from build123d import *

# Parameters (mm, degrees)
SKETCH2_W   = 60
SKETCH2_H   = 60
SKETCH2_W_2 = 50
SKETCH2_H_2 = 50


with BuildPart() as part:
    # Sweep1: sweep along a path in Sketch1
    with BuildLine(Plane.XY) as sweep1_path:
        Line((330, 0), (330, 1500))
        Line((330, 1500), (185.671137026, 1698.283381924))
        Line((185.671137026, 1698.283381924), (0, 1698.283381924))
    # Sketch2 → Sweep1 (sweep)
    with BuildSketch(Plane(origin=(0, 0, 0), x_dir=(1, 0, 0), z_dir=(0, 1, 0))):
        with Locations((330, 0)):
            Rectangle(SKETCH2_W, SKETCH2_H)
        with Locations((330, 0)):
            Rectangle(SKETCH2_W_2, SKETCH2_H_2, mode=Mode.SUBTRACT)
    sweep1 = sweep(path=sweep1_path.line, transition=Transition.RIGHT)

    # Mirror1: Sweep1 across plane
    add(sweep1.mirror(Plane(origin=(0, 0, 0), x_dir=(0, 0, 1), z_dir=(1, 0, 0))))


solid = part.part
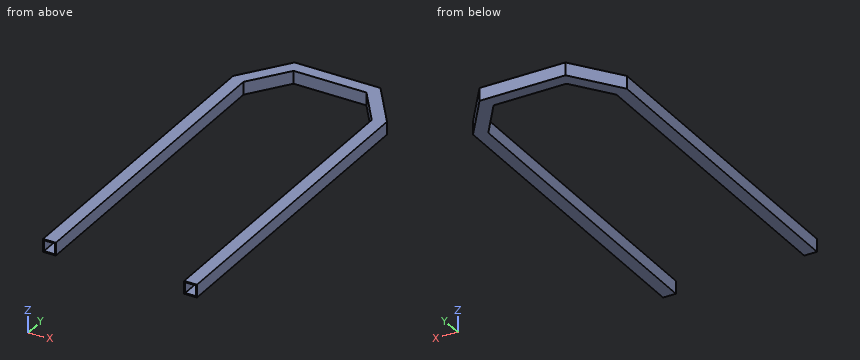
Here's how the part is built. I have some questions about the finished solid (model axes, mm). Round coordinates to 2 decimals unless told otherwise and drop trailing zeros. Write each loop counter-clockwise with the first axis right and the second up, starting at its lowest first coordinate (ties: lowest second). Pieces come first, ordered by that corner, then holes.
1. Suppose I cut it at D-D (x = 256.5). List the corners of the cut face in (y, z) for me, and give its area (3 significant figures).
2. Suppose I cut it at A-A (y = 338). List the corners of the cut face in (x, z) for me, and give its area (3 significant figures).
3. Suppose I cut it at C-C (x = -94). List the corners of the cut face in (y, z) for me, and give its area (3 significant figures).
4. I need wall thicknesses on L1, parallel to X at y = 1018, z = 6.5; L2, parallel to Y at x = -15.5, z = 9.5; L3, parallel to Z at x = 314, y = 1276.5. Which ranges of each line are inside material? Lowest first, please.
5. Suppose I cut it at B-B (z = -6). List the corners of the cut face in (x, y) for me.
6. Will these pins go through, and if not, where does the flat tip stop? pin 1 Ø5 at (x, z) = (-10.5, 2) entering from -Y; pin 2 Ø12 at (x, z) = (-251, 13.5) entering from +Y.
Answer sheet:
1. outline: (1550, -30) - (1651.95, -30) - (1651.95, 30) - (1550, 30) - close; hole (1558.5, -25) - (1643.46, -25) - (1643.46, 25) - (1558.5, 25) - close
1. area: 1,870 mm2
2. outline: (-360, -30) - (-300, -30) - (-300, 30) - (-360, 30) - close; (300, -30) - (360, -30) - (360, 30) - (300, 30) - close; hole (-355, -25) - (-305, -25) - (-305, 25) - (-355, 25) - close; hole (305, -25) - (355, -25) - (355, 25) - (305, 25) - close
2. area: 2,200 mm2
3. outline: (1668.28, -30) - (1728.28, -30) - (1728.28, 30) - (1668.28, 30) - close; hole (1673.28, -25) - (1723.28, -25) - (1723.28, 25) - (1673.28, 25) - close
3. area: 1,100 mm2
4. L1: x = -360 to -355, -305 to -300, 300 to 305, 355 to 360
4. L2: y = 1668.28 to 1673.28, 1723.28 to 1728.28
4. L3: z = -30 to -25, 25 to 30
5. outline: (-360, 0) - (-355, 0) - (-355, 1508.14) - (-198.4, 1723.28) - (198.4, 1723.28) - (355, 1508.14) - (355, 0) - (360, 0) - (360, 1509.76) - (200.94, 1728.28) - (-200.94, 1728.28) - (-360, 1509.76) - close; (-305, 0) - (-300, 0) - (-300, 1490.24) - (-170.4, 1668.28) - (170.4, 1668.28) - (300, 1490.24) - (300, 0) - (305, 0) - (305, 1491.86) - (172.95, 1673.28) - (-172.95, 1673.28) - (-305, 1491.86) - close
6. pin 1: stops at y = 1668.28
6. pin 2: stops at y = 1667.75
